The model under review builds one solid part; all positions refer to its coordinate system, in mm. A direction names the side the tool comes from. Round coordinates to 2 decimals unless told otherwise and drop trailing zeros. Order: outer loops, then holes, each group sorted by start corner. A loop starts at its lowest first (then second) coordinate and runs counter-clockwise, first axis right, second up. Notation, with made-up numbers: (-17, -2.75) -> (-3, -2.75) arc R19 cw to (-3, 2.25) -> close; hole circle Ø1 at (-7, -20). An arc over 180 degrees is marked (long way). Return JSON: item names as keys, results as strings. Group by question number.
from build123d import *

# Parameters (mm, degrees)
SKETCH1_W           = 355.6
SKETCH1_H           = 88.9
BOSS_EXTRUDE1_DEPTH = 9.525
SKETCH2_R           = 3.1623
CUT_EXTRUDE1_DEPTH  = 367.667827366
CUT_EXTRUDE2_DEPTH  = 367.667827366


with BuildPart() as part:
    # Sketch1 → Boss-Extrude1 (new body)
    with BuildSketch(Plane.XY):
        with Locations((177.8, 44.45)):
            Rectangle(SKETCH1_W, SKETCH1_H)
    extrude(amount=BOSS_EXTRUDE1_DEPTH)

    # Sketch2 → Cut-Extrude1 (cut, through all)
    with BuildSketch(Plane.XY.offset(9.525)):
        with Locations((6.35, 76.2)):
            Circle(SKETCH2_R)
        with Locations((6.35, 12.7)):
            Circle(SKETCH2_R)
        with Locations((349.25, 76.2)):
            Circle(SKETCH2_R)
        with Locations((349.25, 12.7)):
            Circle(SKETCH2_R)
    extrude(amount=-CUT_EXTRUDE1_DEPTH, mode=Mode.SUBTRACT)

    # Sketch3 → Cut-Extrude2 (cut, through all)
    with BuildSketch(Plane.XY.offset(9.525)):
        with BuildLine():
            Line((25.4, 71.755), (330.2, 71.755))
            ThreePointArc((330.2, 71.755), (338.455, 63.5), (330.2, 55.245))
            Line((330.2, 55.245), (25.4, 55.245))
            ThreePointArc((25.4, 55.245), (17.145, 63.5), (25.4, 71.755))
        make_face()
    extrude(amount=-CUT_EXTRUDE2_DEPTH, mode=Mode.SUBTRACT)


solid = part.part
Item 1: Consider section C-C on y = 63.5. State the section outline as (x, z) points (3 decimals).
Item 2: Consider section D-D on x = 126. State the section outline as (y, z) points (3 decimals).
Item 3: Consider section A-A on x = 6.35. State the section outline as (y, z) points (3 decimals), plus the area to 3 significant figures.
Item 4: The part is to be moulded in two halves that separate along Y. For faces 1 (the face through (175, 0, 5)), 2 (the face through (175, 45, 9.525)), 3 (the face through (175, 88.9, 5)), 4 (the face through (5.664, 73.113, 4.829)), say which applies: +Y half, -Y half, draft (parallel to the pull), parting line (faces both ways), or undercut.
Item 5: Wall thickness on line 1 along Y through (x, z) = (349.25, 4.5); line 2 along Y through (x, z) = (249, 2.5) (3 decimals); line 3 along X through (y, z) = (64, 5): over which ranges is each line inside the solid? List them lowest first.
Item 6: Consider section B-B on z = 2.25. State the section outline as (x, y) points (3 decimals), plus the area to 3 significant figures.
Item 7: For faces 5 (the face through (338.453, 63.682, 4.829)), 6 (the face through (355.6, 44, 5)), list the 3-axis set-ups (+Z, -Z, +X, -X, +Y, -Y) from which the entire face can be reached by the end or side of a thin tool; tool diameter is ignored.
Values:
{
 "1": {"outline": "(0, 0) -> (17.145, 0) -> (17.145, 9.525) -> (0, 9.525) -> close; (338.455, 0) -> (355.6, 0) -> (355.6, 9.525) -> (338.455, 9.525) -> close"},
 "2": {"outline": "(0, 0) -> (55.245, 0) -> (55.245, 9.525) -> (0, 9.525) -> close; (71.755, 0) -> (88.9, 0) -> (88.9, 9.525) -> (71.755, 9.525) -> close"},
 "3": {"outline": "(0, 0) -> (9.538, 0) -> (9.538, 9.525) -> (0, 9.525) -> close; (15.862, 0) -> (73.038, 0) -> (73.038, 9.525) -> (15.862, 9.525) -> close; (79.362, 0) -> (88.9, 0) -> (88.9, 9.525) -> (79.362, 9.525) -> close", "area": "726 mm^2"},
 "4": {"face 1": "-Y half", "face 2": "draft", "face 3": "+Y half", "face 4": "undercut"},
 "5": {"line 1": "0 to 9.54, 15.86 to 73.04, 79.36 to 88.9", "line 2": "0 to 55.245, 71.755 to 88.9", "line 3": "0 to 17.16, 338.44 to 355.6"},
 "6": {"outline": "(0, 0) -> (355.6, 0) -> (355.6, 88.9) -> (0, 88.9) -> close; hole circle Ø6.325 at (6.35, 12.7); hole circle Ø6.325 at (6.35, 76.2); hole (25.4, 55.245) -> (330.2, 55.245) arc R8.255 ccw to (330.2, 71.755) -> (25.4, 71.755) arc R8.255 ccw to start; hole circle Ø6.325 at (349.25, 12.7); hole circle Ø6.325 at (349.25, 76.2)", "area": "26,200 mm^2"},
 "7": {"face 5": "+Z, -Z", "face 6": "+Z, -Z, +X, +Y, -Y"}
}
